The listing builds one solid part. Answer for the finished solid, in the listing's coordinates (mm). Face numbers are marked on the shaded views. Give positions to 0.01 mm unless a question says otherwise; leave off trailing zeros. Loops run counter-clockwise (first coordinate to the right, second up) from the corner with the lowest first, then second, coordinate; pieces in that order, holes last. Notation, with made-up numbers: M 24,85 L 30,85 A26 cw 30,112 Z; hole C 59.5,46 d7. An arc over 180 degrees is marked long. Use one line per item in the form item = value. Start each with the question number.
1. Each of these flat-tipped pins is pushed along its axis until it touches: pin 1 Ø9 at (x, y) = (47.5, -58.5) entering from +Z; pin 2 Ø4.5 at (y, z) = (-8, 1.5) entering from -X; pin 3 Ø1.5 at (x, z) = (-31, 13.5) entering from +Y. Where does it stop, or does it pass through?
2. The part is cut by section B-B (y = 21). Write down the section's boundary in (x, z).
3. The part is cut by section C-C (x = 14). Write down the section's boundary in (y, z).
4. The part is cut by section A-A (z = 10). Write down the section's boundary in (x, y), and give its area (3 significant figures).
5. The mould has two halves that part along Y. Classify the marked faces 1, 2 and 3: released by +Y, released by -Y, zero draft, split by the parting line, or undercut.
6. The part is cut by section D-D (z = 2.25). Write down the section's boundary in (x, y).
7. Straight lines are drawn through the part: line 1 (Y direction, x = 46, z = 5.75); line 2 (Y direction, x = -46, z = 3.75); line 3 (X direction, y = -40.5, z = 3.25). For each, find the intervals that lie inside material, in ascending order. Write a range as from..to.
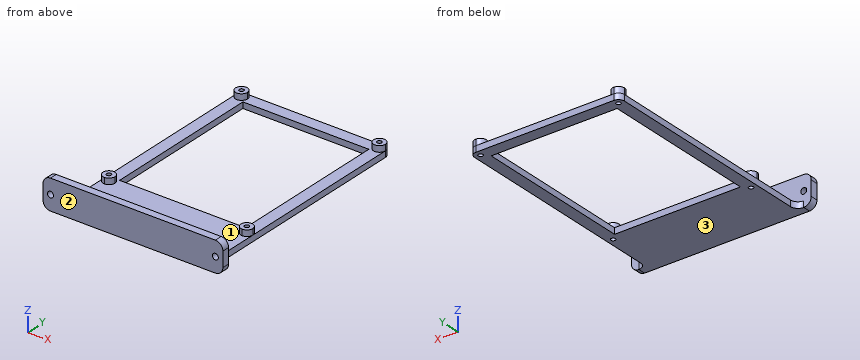
from build123d import *

# Parameters (mm, degrees)
F0_W      = 100
F0_H      = 122.999
F0_R      = 1.5
F0_W_2    = 84
F0_H_2    = 106.999
F1_DEPTH  = 4
F2_R      = 1.5
F3_DEPTH  = 4
F4_W      = 100
F4_H      = 4
F5_DEPTH  = 30
F7_DEPTH  = 20
F8_R      = 4.99999
F9_R      = 3.9999
F10_R     = 2
F11_DEPTH = 10


# Not quite as in the source:
# - a fillet or chamfer is up to 0.001 mm smaller than in the source, because OpenCascade refuses the exact size


with BuildPart() as f1:
    # F0 (on Top) → F1 (new body)
    with BuildSketch(Plane.XY):
        Rectangle(F0_W, F0_H)
        with Locations((-46, -57.4995)):
            Circle(F0_R, mode=Mode.SUBTRACT)
        with Locations((46, -57.4995)):
            Circle(F0_R, mode=Mode.SUBTRACT)
        with Locations((-46, 57.4995)):
            Circle(F0_R, mode=Mode.SUBTRACT)
        Rectangle(F0_W_2, F0_H_2, mode=Mode.SUBTRACT)
        with Locations((46, 57.4995)):
            Circle(F0_R, mode=Mode.SUBTRACT)
    extrude(amount=F1_DEPTH)

    # F2 (on face) → F3 (join)
    with BuildSketch(Plane.XY.offset(4)):
        with BuildLine():
            ThreePointArc((-42, 57.4995), (-43.1715728523, 60.3279271017), (-45.999999935, 61.4995))
            ThreePointArc((-45.999999935, 61.4995), (-48.8284271017, 60.3279271477), (-50, 57.4995))
            ThreePointArc((-50, 57.4995), (-46, 53.4995), (-42, 57.4995))
        make_face()
        with Locations((-46, 57.4995)):
            Circle(F2_R, mode=Mode.SUBTRACT)
        with BuildLine():
            ThreePointArc((46, 61.4995), (43.1715728753, 54.6710728753), (50, 57.4995))
            ThreePointArc((50, 57.4995), (48.8284271247, 60.3279271247), (46, 61.4995))
        make_face()
        with Locations((46, 57.4995)):
            Circle(F2_R, mode=Mode.SUBTRACT)
        with BuildLine():
            ThreePointArc((45.9999999936, -61.4995), (48.8284271225, -60.327927127), (50, -57.4995))
            ThreePointArc((50, -57.4995), (43.1715728775, -54.671072873), (45.9999999936, -61.4995))
        make_face()
        with Locations((46, -57.4995)):
            Circle(F2_R, mode=Mode.SUBTRACT)
        with BuildLine():
            ThreePointArc((-50, -57.4995), (-48.8284271247, -60.3279271247), (-46, -61.4995))
            ThreePointArc((-46, -61.4995), (-43.1715728753, -60.3279271247), (-42, -57.4995))
            ThreePointArc((-42, -57.4995), (-46, -53.4995), (-50, -57.4995))
        make_face()
        with Locations((-46, -57.4995)):
            Circle(F2_R, mode=Mode.SUBTRACT)
    extrude(amount=F3_DEPTH)

    # F4 (on face) → F5 (join)
    with BuildSketch(Plane.XZ.offset(61.4995)):
        with Locations((0, 2)):
            Rectangle(F4_W, F4_H)
    extrude(amount=F5_DEPTH)

    # F6 (on face) → F7 (join)
    with BuildSketch(Plane(origin=(0, 0, 0), x_dir=(1, 0, 0), z_dir=(0, 0, -1))):
        Polygon((50, 91.4995), (60, 91.4995), (60, 96.4995), (-50, 96.4995), (-60, 96.4995), (-60, 91.4995), (-50, 91.4995), align=None)
    extrude(amount=-F7_DEPTH)

    # F8 (radius 5 in the source; OpenCascade refuses exactly that, so slightly less here)
    f8_edges = [f1.edges().sort_by_distance(p)[0] for p in [
        (-60, -93.9995, 20),
        (-60, -93.9995, 0),
        (60, -93.9995, 0),
        (60, -93.9995, 20),
        (50, -91.4995, 2),
        (-50, -91.4995, 2),
    ]]
    fillet(f8_edges, radius=F8_R)

    # F9 (radius 4 in the source; OpenCascade refuses exactly that, so slightly less here)
    f9_edges = [f1.edges().sort_by_distance(p)[0] for p in [
        (50, 61.4995, 2),
        (-50, 61.4995, 2),
    ]]
    fillet(f9_edges, radius=F9_R)

    # F10 (on face) → F11 (cut)
    with BuildSketch(Plane(origin=(0, -91.4995, 0), x_dir=(-1, 0, 0), z_dir=(0, 1, 0))):
        with Locations((55, 10)):
            Circle(F10_R)
        with Locations((-55, 10)):
            Circle(F10_R)
    extrude(amount=-F11_DEPTH, mode=Mode.SUBTRACT)


solid = f1.part
Derived:
q1.pin_1 = 8
q1.pin_2 = -50
q1.pin_3 = -91.5
q2.outline = M -50,0 L -42,0 L -42,4 L -50,4 Z; M 42,0 L 50,0 L 50,4 L 42,4 Z
q3.outline = M -96.5,0 L -53.5,0 L -53.5,4 L -91.5,4 L -91.5,20 L -96.5,20 Z; M 53.5,0 L 61.5,0 L 61.5,4 L 53.5,4 Z
q4.outline = M -60,-96.5 L -57,-96.5 L -57,-91.5 L -60,-91.5 Z; M -53,-96.5 L 53,-96.5 L 53,-91.5 L -53,-91.5 Z; M 57,-96.5 L 60,-96.5 L 60,-91.5 L 57,-91.5 Z
q4.area = 560 mm2
q5.face_1 = undercut
q5.face_2 = released by -Y
q5.face_3 = zero draft
q6.outline = M -59.18,-96.5 L 59.18,-96.5 L 59.18,-91.5 L 55,-91.5 A5 cw 50,-86.5 L 50,57.5 A4 ccw 46,61.5 L -46,61.5 A4 ccw -50,57.5 L -50,-86.5 A5 cw -55,-91.5 L -59.18,-91.5 Z; hole C -46,-57.5 d3; hole C -46,57.5 d3; hole M -42,-53.5 L 42,-53.5 L 42,53.5 L -42,53.5 Z; hole C 46,-57.5 d3; hole C 46,57.5 d3
q7.line_1 = -96.5..-91.5, -61.5..-59, -56..-53.5, 53.5..56, 59..61.5
q7.line_2 = -96.5..-59, -56..56, 59..61.5
q7.line_3 = -50..-42, 42..50
